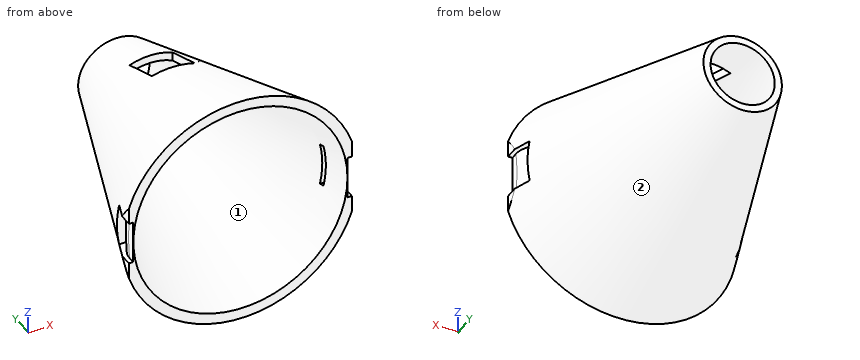
Autodesk Inventor part; units mm, degrees
ref_plane "YZ Plane" through (0, 0, 0) normal (1, 0, 0) x (0, 1, 0)
ref_plane "XZ Plane" through (0, 0, 0) normal (0, 1, 0) x (-1, 0, 0)
ref_plane "XY Plane" through (0, 0, 0) normal (0, 0, 1) x (1, 0, 0)
sketch "Sketch1" plane through (0, 0, 0) normal (0, 1, 0) x (-1, 0, 0)
  point P0 (0, 0)
sketch "Sketch2" plane through (0, 0, 0) normal (0, 1, 0) x (-1, 0, 0)
  circle A0 centre (0, 0) radius 7.5
  dimension "d0" = 15
extrude "Extrusion1" add sketch "Sketch2" along normal blind 60
sketch "Sketch3" plane through (0, 60, 0) normal (0, 1, 0) x (1, 0, 0)
  circle A0 centre (0, 0) radius 7.5
sketch "Sketch4" plane through (0, 0, 0) normal (0, -1, 0) x (1, 0, 0)
  circle A0 centre (0, 0) radius 25
  circle A1 centre (0, 0) radius 7.5
  circle A2 centre (0, 0) radius 27.5
  dimension "d3" = 50
  dimension "d4" = 55
loft "Loft1" add profiles "Sketch4" section 1 edges at (7.5, 60, 0) contours A0 | A1 | A2
sketch "Sketch5" plane through (0, 0, 0) normal (0, -1, 0) x (1, 0, 0)
  circle A0 centre (0, 0) radius 7.5
  circle A1 centre (0, 0) radius 27.5
  circle A2 centre (0, 0) radius 25
  circle A3 centre (0, 0) radius 7.5
  dimension "d9" = 50
  dimension "d10" = 15
sketch "Sketch6" plane through (0, 60, 0) normal (0, 1, 0) x (1, 0, 0)
  circle A0 centre (0, 0) radius 7.5
extrude "Extrusion2" cut sketch "Sketch6" against normal blind 5
sketch "Sketch7" plane through (0, 55, 0) normal (0, 1, 0) x (1, 0, 0)
  circle A0 centre (0, 0) radius 7.5
  line L0 (-11.197, -10.4421) -> (10.2744, -10.4421)
  line L1 (10.2744, -10.4421) -> (10.2744, 11.5325)
  line L2 (10.2744, 11.5325) -> (-11.197, 11.5325)
  line L3 (-11.197, 11.5325) -> (-11.197, -10.4421)
loft "Loft2" cut profiles "Sketch5" section 1 edges at (-7.5, 55, 0) contours A0 | A2
extrude "Extrusion3" cut sketch "Sketch7" along normal through all
sketch "Sketch8" plane through (0, 0, 0) normal (0, -1, 0) x (1, 0, 0)
  circle A0 centre (0, 0) radius 25
  circle A1 centre (0, 0) radius 27.5
  line L0 (27.5, 0) -> (27.5, -5)
  line L1 (27.0416, -5) -> (26.0416, -5)
  line L2 (26.0416, -5) -> (26.0416, 5)
  line L3 (26.0416, 5) -> (27.0416, 5)
  line L4 (27.0416, 5) -> (27.0416, -5)
  line L5 (-27.5, 0) -> (-27.5, -5)
  line L6 (-27.0416, -5) -> (-26.0416, -5)
  line L7 (-26.0416, -5) -> (-26.0416, 5)
  line L8 (-26.0416, 5) -> (-27.0416, 5)
  line L9 (-27.0416, 5) -> (-27.0416, -5)
  line L10 (26.0416, -5) -> (25.0416, -5)
  line L11 (25.0416, -5) -> (25.0416, 5)
  line L12 (25.0416, 5) -> (26.0416, 5)
  line L13 (26.0416, 5) -> (26.0416, -5)
  line L14 (-26.0416, -5) -> (-25.0416, -5)
  line L15 (-25.0416, -5) -> (-25.0416, 5)
  line L16 (-25.0416, 5) -> (-26.0416, 5)
  line L17 (-26.0416, 5) -> (-26.0416, -5)
  line L18 (-26.0416, 5) -> (-26.0416, 8.8365)
  line L19 (-26.0416, -5) -> (-26.0416, -8.8365)
  line L20 (26.0416, -5) -> (26.0416, -8.8365)
  line L21 (26.0416, 5) -> (26.0416, 8.8365)
  circle A2 centre (0, 0) radius 27.5
  dimension "d19" = 5
  dimension "d20" = 1
  dimension "d21" = 10
  dimension "d22" = 5
  dimension "d23" = 1
  dimension "d24" = 10
  dimension "d25" = 1
  dimension "d26" = 1
extrude "Extrusion4" cut sketch "Sketch8" against normal through all contours A1 L4 | L3 L21 A1 | L4 L1 L2 L3 | A1 L20 L1 | L18 L8 A1 | A1 L6 L19 | L9 A1 | L8 L7 L6 L9
sketch "Sketch9" plane through (0, 0, 0) normal (0, -1, 0) x (1, 0, 0)
  circle A0 centre (0, 0) radius 27.5
  circle A1 centre (0, 0) radius 25
  line L0 (27.5, 0) -> (27.5, -5)
  line L1 (26.0416, -8.8365) -> (26.0416, 8.8365)
  line L2 (27.0416, -5) -> (26.0416, -5)
  line L3 (26.0416, -5) -> (26.0416, 5)
  line L4 (26.0416, 5) -> (27.0416, 5)
  line L5 (27.0416, 5) -> (27.0416, -5)
  line L6 (26.0416, 5) -> (25.0416, 5)
  line L7 (25.0416, 5) -> (25.0416, -5)
  line L8 (25.0416, -5) -> (26.0416, -5)
  line L9 (26.0416, -5) -> (26.0416, 5)
  line L10 (-27.5, 0) -> (-27.5, -5)
  line L11 (-26.0416, 8.8365) -> (-26.0416, -8.8365)
  line L12 (-27.0416, -5) -> (-26.0416, -5)
  line L13 (-26.0416, -5) -> (-26.0416, 5)
  line L14 (-26.0416, 5) -> (-27.0416, 5)
  line L15 (-27.0416, 5) -> (-27.0416, -5)
  line L16 (-26.0416, -5) -> (-25.0416, -5)
  line L17 (-25.0416, -5) -> (-25.0416, 5)
  line L18 (-25.0416, 5) -> (-26.0416, 5)
  line L19 (-26.0416, 5) -> (-26.0416, -5)
  dimension "d29" = 5
  dimension "d30" = 10
  dimension "d31" = 1
  dimension "d32" = 5
  dimension "d33" = 10
  dimension "d34" = 1
extrude "Extrusion5" cut sketch "Sketch9" against normal blind 7 contours L1 L8 L7 L6 | L18 L17 L16 L11
sketch "Sketch10" plane through (25.0416, 0, 5) normal (1, 0, 0) x (0, 0, -1)
  line L0 (0, 0) -> (10, 0)
  line L1 (10, 0) -> (10, 7)
  line L2 (10, 7) -> (0, 7)
  line L3 (0, 7) -> (0, 0)
  line L4 (10, 7) -> (0, 7)
  line L5 (0, 7) -> (0, 6)
  line L6 (0, 6) -> (10, 6)
  line L7 (10, 6) -> (10, 7)
  point P0 (5, 0)
  dimension "d37" = 10
  dimension "d38" = 7
  dimension "d39" = 1
extrude "Extrusion6" cut sketch "Sketch10" against normal through all contours L3 L2 L1 L6
fillet "Fillet1" radius 5 1 edges at (25.0416, 6, 0)
fillet "Fillet2" radius 5 1 edges at (-25.0416, 6, 0)
sketch "Sketch11" plane through (0, 0, 0) normal (0, -1, 0) x (1, 0, 0)
  line L0 (0, 0) -> (35, 0)
  line L1 (35, 0) -> (-35, 0)
  line L2 (-35, 0) -> (-35, 30)
  line L3 (-35, 30) -> (35, 30)
  line L4 (35, 30) -> (35, 0)
  line L5 (0, 30) -> (5, 30)
  line L6 (5, 30) -> (-5, 30)
  line L7 (-5, 30) -> (-5, 40)
  line L8 (-5, 40) -> (5, 40)
  line L9 (5, 40) -> (5, 30)
  dimension "d44" = 35
  dimension "d45" = 70
  dimension "d46" = 30
  dimension "d47" = 5
  dimension "d48" = 10
  dimension "d49" = 10
extrude "Extrusion7" add sketch "Sketch11" against normal blind 50 contours L3 L7 L8 L9
sketch "Sketch12" plane through (5, 0, 40) normal (1, 0, 0) x (0, 0, -1)
  line L0 (10, 0) -> (10, 50)
  line L1 (10, 0) -> (10, 35)
  line L2 (10, 35) -> (0, 35)
  line L3 (0, 0) -> (0, 50)
  point P0 (40, 0)
  dimension "d52" = 35
sketch "Sketch13" plane through (5, 0, 30) normal (0, 0, -1) x (-1, 0, 0)
  point P0 (5, 0)
sketch "Sketch14" plane through (-5, 0, 40) normal (0, 0, 1) x (1, 0, 0)
  line L0 (10, 0) -> (10, 50)
  line L1 (10, 35) -> (10, 40)
  line L2 (0, 0) -> (0, 50)
  line L3 (10, 40) -> (0, 40)
  line L4 (0, 40) -> (0, 30)
  line L5 (0, 30) -> (10, 30)
  line L6 (10, 30) -> (10, 40)
  point P0 (5, 0)
  dimension "d53" = 5
  dimension "d54" = 10
extrude "Extrusion8" cut sketch "Sketch14" against normal blind 35
sketch "Sketch15" plane through (0, 50, 0) normal (0, 1, 0) x (1, 0, 0)
  line L0 (5, -30) -> (-5, -30)
  line L1 (-5, -40) -> (5, -40)
  line L2 (-5, -30) -> (5, -30)
  line L3 (5, -30) -> (5, -40)
  line L4 (5, -40) -> (-5, -40)
  line L5 (-5, -40) -> (-5, -30)
  point P0 (0, 0)
extrude "Extrusion9" cut sketch "Sketch15" against normal through all
properties part number "cone_p3_testpart1_3DPrint"
The listing builds one solid part. Answer for the finished solid, in the listing's coordinates (mm). Face numbers are marked on the shaded views. Give positions to 0.01 mm unless a question says otherwise; leave off trailing zeros. Loops run counter-clockwise (first coordinate to the right, second up) from the corner with the lowest first, then second, coordinate; pieces in that order, holes last. Notation, with made-up numbers: (86.25, 89.5) - (116.25, 89.5) arc R11 ccw to (116.25, 98.5) - close; hole circle Ø5 at (13.25, -4.5). An arc over 180 degrees is marked (long way). Answer as CSV lines item,"result". Start each with the question number.
Item 1: A cutting plane is placed at B-B on z = 0. Count the separate pieces of the cut face and the enclosed holes in it, then the cut area to 3 significant figures.
Item 2: A cutting plane is placed at A-A on x = 0. Determine the outline of the cut face in (y, z).
Item 3: A cutting plane is placed at D-D on y = 33. Determine the outline of the cut face in (x, z), then the cut area to 3 significant figures.
Item 4: A cutting plane is placed at C-C on y = 44.5. Determine the outline of the cut face in (x, z).
Item 5: The mould has two halves that part along Z. Classify the marked faces 1 and 2: +Z half, -Z half, draft (parallel to the pull), parting line (faces both ways), or undercut.
Item 6: Each of these flat-tipped pins is pushed along its axis until it touches: pin 1 (1.6 mm diameter, centred on y = 1, z = -2, fed in from -X); pin 2 (10 mm diameter, centred on x = -10, y = 33, fed in from -Z); pin 3 (8 mm diameter, centred on x = 1.5, y = 11.5, fed in from +Z). Where does it stop, or does it pass through?
Item 7: Find the intervals of material crossed by line 1 (Z direction, x = -11, y = 33.5); line 2 (X direction, y = 3, z = -6.5); line 3 (X direction, y = 40, z = 8.5), in increasing order. Write a range as from..to.
Found:
1,separate pieces,"4"
1,enclosed holes,"0"
1,area,"202 mm^2"
2,outline,"(0, -27.5) - (55, -9.17) - (55, -7.5) - (0, -25) - close; (0, 25) - (30, 15.45) - (30, 17.5) - (0, 27.5) - close; (40, 12.27) - (55, 7.5) - (55, 9.17) - (40, 14.17) - close"
3,outline,"(-5, 13.61) - (-5, 15.72) arc R16.5 ccw (long way) to (5, 15.72) - (5, 13.61) arc R14.5 cw (long way) to start"
3,area,"174 mm^2"
4,outline,"circle Ø25.33 at (0, 0); hole circle Ø21.68 at (0, 0)"
5,face 1,"undercut"
5,face 2,"parting line"
6,pin 1,"stops at x = -25.04"
6,pin 2,"stops at z = -16.46"
6,pin 3,"stops at z = 24.97"
7,line 1,"z = -12.07..-9.2, 9.2..12.07"
7,line 2,"x = -25.69..-23.15, 23.15..25.69"
7,line 3,"x = -11.33..-8.85, 8.85..11.33"
